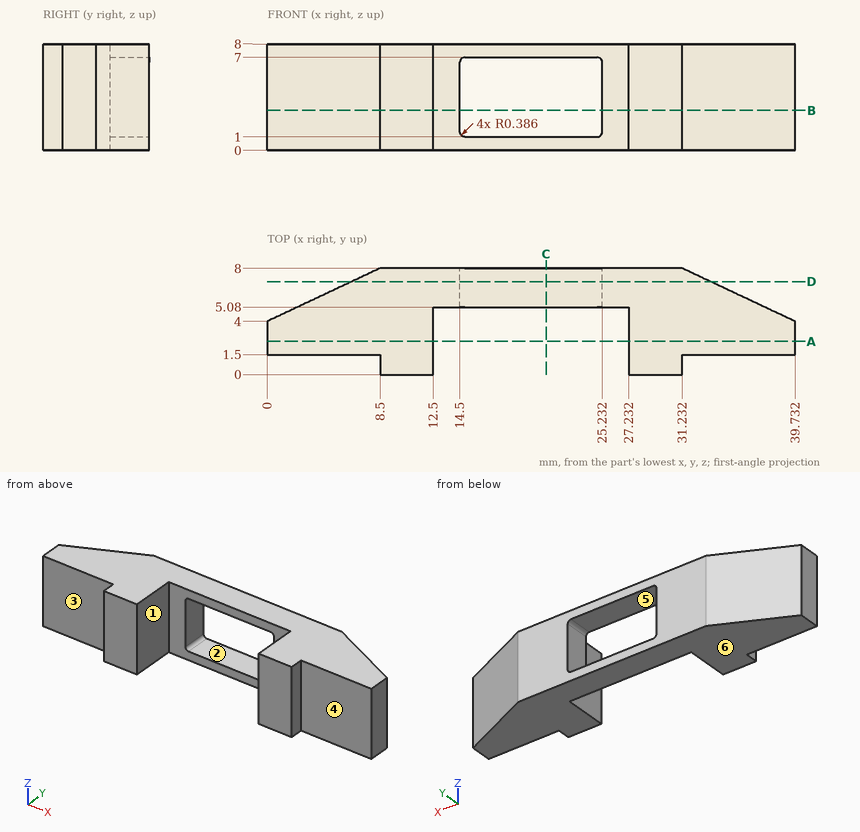
For this review, use the dimensioned drawing (mm, ordinates from the lowest corner) and the shaded views. A direction names the side the tool comes from. Round coordinates to 2 decimals unless told otherwise and drop trailing zeros. Order: outer loops, then holes, each group sorted by start corner. A loop starts at its lowest first (then second) coordinate and runs counter-clockwise, first axis right, second up. Notation, with made-up numbers: (76.5, 12) -> (98.5, 12) arc R26 cw to (98.5, 34) -> close; hole circle Ø11 at (-37.75, 84). An arc over 180 degrees is marked (long way). Use CSV: the item, a comma, the result in double quotes. Start each with the question number.
(1) Mouldability with a two-part tool opening along Z and no side actions: class the marked faces 4, 5 and 6 as pulls with the +Z half, pulls with the -Z half, needs draft (parallel to the pull), parting line crosses it, or undercut.
(2) Consider section C-C on x = 21. Write out the cut boundary in (y, z).
(3) Wall thickness on probe 1 along X at (y, z) = (2.5, 7.75); probe 2 along X at (y, z) = (0.75, 4.75); probe 3 along Z at (x, y) = (21.5, 6): over which ranges is each line inside the solid? List them lowest first. Write a range as from..to.
(4) Consider section A-A on y = 2.5. Write out the cut boundary in (x, z).
(5) Insertion check: pin 1 (1.6 mm diameter, centred on y = 0.5, z = 3, fed in from -X); pin 2 (4 mm diameter, centred on x = 19.5, z = 3.5, fed in from -Y); pin 3 (4 mm diameter, centred on x = 35, z = 5.5, fed in from -Y); pin 4 (0.9 mm diameter, centred on y = 6, z = 2.5, fed in from +X). Each pin has a flat end and moves straight along its axis. Give the tip position at first contact, or say it passes through.
(6) Tool access review of the marked faces 1, 2 and 3: name each direction out of +Z, -Z, +X, -X, +Y, -Y from which nothing blocks a thin tool from reaching the whole face with its end or side.
(7) Consider section D-D on y = 7. Write out the cut boundary in (x, z) (1 decimal).
(8) Consider section B-B on z = 3. Write out the cut boundary in (x, y), and give its area (3 significant figures).
Responses:
1,face 4,"needs draft"
1,face 5,"undercut"
1,face 6,"pulls with the -Z half"
2,outline,"(5.08, 0) -> (8, 0) -> (8, 1) -> (5.08, 1) -> close; (5.08, 7) -> (8, 7) -> (8, 8) -> (5.08, 8) -> close"
3,probe 1,"0..12.5, 27.23..39.73"
3,probe 2,"8.5..12.5, 27.23..31.23"
3,probe 3,"0..1, 7..8"
4,outline,"(0, 0) -> (12.5, 0) -> (12.5, 8) -> (0, 8) -> close; (27.23, 0) -> (39.73, 0) -> (39.73, 8) -> (27.23, 8) -> close"
5,pin 1,"x = 8.5"
5,pin 2,"through"
5,pin 3,"y = 1.5"
5,pin 4,"x = 36.44"
6,face 1,"+Z, -Z, -Y"
6,face 2,"+Y, -Y"
6,face 3,"+Z, -Z, -X, -Y"
7,outline,"(6.4, 0) -> (33.4, 0) -> (33.4, 8) -> (6.4, 8) -> close; hole (14.5, 1.4) arc R0.4 ccw to (14.9, 1) -> (24.8, 1) arc R0.4 ccw to (25.2, 1.4) -> (25.2, 6.6) arc R0.4 ccw to (24.8, 7) -> (14.9, 7) arc R0.4 ccw to (14.5, 6.6) -> close"
8,outline,"(0, 1.5) -> (8.5, 1.5) -> (8.5, 0) -> (12.5, 0) -> (12.5, 5.08) -> (14.5, 5.08) -> (14.5, 8) -> (8.5, 8) -> (0, 4) -> close; (25.23, 5.08) -> (27.23, 5.08) -> (27.23, 0) -> (31.23, 0) -> (31.23, 1.5) -> (39.73, 1.5) -> (39.73, 4) -> (31.23, 8) -> (25.23, 8) -> close"
8,area,"152 mm²"
